Check sheet for the modelled part. Datum: model origin and axes. Units: mm. A direction names the side the tool comes from. Round coordinates to 2 decimals unless told otherwise and drop trailing zeros. Loops run counter-clockwise (first coordinate to the right, second up) from the corner with the lowest first, then second, coordinate; pieces in that order, holes last. Notation, with made-up numbers: M 24,-14.75 L 70,-14.75 A30 cw 70,13.25 Z; hole C 47,-5 d9. An arc over 180 degrees is marked long. Write item = value, one per line. Start each with the question number.
(1) Cross-section at A-A on y = 22. Record the boundary of the cut face in (x, z).
(2) Mould release check, pull along X, two halves, no side actions. Record for faces 5 (the face through (74, 1, 2)), 6 (the face through (-1, 30, 15)), 7 (the face through (82.457, 5.916, 15.931)), 8 (the face through (-87.63, 4.23, 27.82)): pulls with the +X half, pulls with the -X half, needs draft (parallel to the pull), parting line crosses it, or undercut.
(3) Scan lines: L1, parallel to Z at x = -79.5, y = 5.5; L2, parallel to Y at x = -3.5, z = 7.5; L3, parallel to Y at x = -78.5, z = 24.5. Record each from-to range of solid material in increasing order. Write a range as from..to.
(4) Cross-section at B-B on x = -79.5. Record the boundary of the cut face in (y, z), plus the area to 3 significant figures.
(5) Set-up check for faces 1 (the face through (-87.07, 10.5, 15.14)), 2 (the face through (-57.07, 28.5, 15.14)), 3 (the face through (70.5, 27, 15)), 4 (the face through (79, 11, 28)): record each of +Z, -Z, +X, -X, +Y, -Y from which the full face is reachable in a straight line by a thin tool's end or side.
(6) Cross-section at C-C on z = 15. Record the boundary of the cut face in (x, y), plus the area to 3 significant figures.
(7) Go/stop test with flat-tipped pins: P1, Ø8, axis at y = 31.5, z = 11, coming from the +X side; P2, Ø10, axis at y = 11.5, z = 19.5, coming from the -X side; P3, Ø10, axis at x = 79.5, z = 15, coming from the +Y side; P4, Ø9, axis at x = 81, z = 11, coming from the +Y side. Record where each tip stops, or that it passes through.
(8) Cross-section at D-D on x = 33.5. Record the boundary of the cut face in (y, z).
from build123d import *

# Parameters (mm, degrees)
F1_DEPTH = 30
F2_R     = 5
F3_R     = 3.1
F4_DEPTH = 25


with BuildPart() as f1:
    # F0 (on Top) → F1 (new body)
    with BuildSketch(Plane.XY):
        Polygon((-88.5, 12), (-88.5, 0), (-58.5, 0), (-58.5, 30), (58.5, 30), (58.5, 0), (88.5, 0), (88.5, 12), (70.5, 12), (70.5, 42), (-70.5, 42), (-70.5, 12), align=None)
    extrude(amount=F1_DEPTH)

    # F2
    f2_edges = [f1.edges().sort_by_distance(p)[0] for p in [
        (70.5, 42, 15),
        (-70.5, 42, 15),
        (0, 42, 0),
        (0, 42, 30),
        (-88.5, 6, 30),
        (-73.5, 0, 30),
        (-58.5, 15, 30),
        (0, 30, 30),
        (58.5, 15, 30),
        (73.5, 0, 30),
        (88.5, 6, 30),
        (79.5, 12, 30),
        (70.5, 27, 30),
        (-70.5, 27, 30),
        (-79.5, 12, 30),
        (-88.5, 6, 0),
        (-73.5, 0, 0),
        (-58.5, 15, 0),
        (0, 30, 0),
        (58.5, 15, 0),
        (73.5, 0, 0),
        (88.5, 6, 0),
        (79.5, 12, 0),
        (70.5, 27, 0),
        (-70.5, 27, 0),
        (-79.5, 12, 0),
        (70.5, 12, 15),
        (-70.5, 12, 15),
        (-58.5, 30, 15),
        (58.5, 30, 15),
        (-88.5, 12, 15),
        (88.5, 12, 15),
    ]]
    fillet(f2_edges, radius=F2_R)

    # F3 (on face) → F4 (cut)
    with BuildSketch(Plane.XZ):
        with Locations((79.5, 15)):
            Circle(F3_R)
        with Locations((-79.5, 15)):
            Circle(F3_R)
    extrude(amount=-F4_DEPTH, mode=Mode.SUBTRACT)


solid = f1.part
Result:
q1.outline = M -70.5,5 A5 ccw -65.5,0 L -63.5,0 A5 ccw -58.5,5 L -58.5,25 A5 ccw -63.5,30 L -65.5,30 A5 ccw -70.5,25 Z; M 58.5,5 A5 ccw 63.5,0 L 65.5,0 A5 ccw 70.5,5 L 70.5,25 A5 ccw 65.5,30 L 63.5,30 A5 ccw 58.5,25 Z
q2.face_5 = needs draft
q2.face_6 = undercut
q2.face_7 = undercut
q2.face_8 = pulls with the -X half
q3.L1 = 0..11.9, 18.1..30
q3.L2 = 30..42
q3.L3 = 0..12
q4.outline = M 0,5 A5 ccw 5,0 L 7,0 A5 ccw 12,5 L 12,11.9 L 0,11.9 Z; M 0,18.1 L 12,18.1 L 12,25 A5 ccw 7,30 L 5,30 A5 ccw 0,25 Z
q4.area = 264 mm^2
q5.face_1 = +Z, -Z, -X, +Y
q5.face_2 = +Z, -Z, -Y
q5.face_3 = +Z, -Z, +X, +Y
q5.face_4 = +Z, +X, +Y
q6.outline = M -88.5,0 L -82.6,0 L -82.6,12 L -83.5,12 A5 ccw -88.5,7 Z; M -76.4,0 L -58.5,0 L -58.5,25 A5 cw -53.5,30 L 53.5,30 A5 cw 58.5,25 L 58.5,0 L 76.4,0 L 76.4,12 L 75.5,12 A5 cw 70.5,17 L 70.5,37 A5 ccw 65.5,42 L -65.5,42 A5 ccw -70.5,37 L -70.5,17 A5 cw -75.5,12 L -76.4,12 Z; M 82.6,0 L 88.5,0 L 88.5,7 A5 ccw 83.5,12 L 82.6,12 Z
q6.area = 2,700 mm^2
q7.P1 = 70.5
q7.P2 = -88.5
q7.P3 = 12.1
q7.P4 = 12
q8.outline = M 30,5 A5 ccw 35,0 L 37,0 A5 ccw 42,5 L 42,25 A5 ccw 37,30 L 35,30 A5 ccw 30,25 Z
